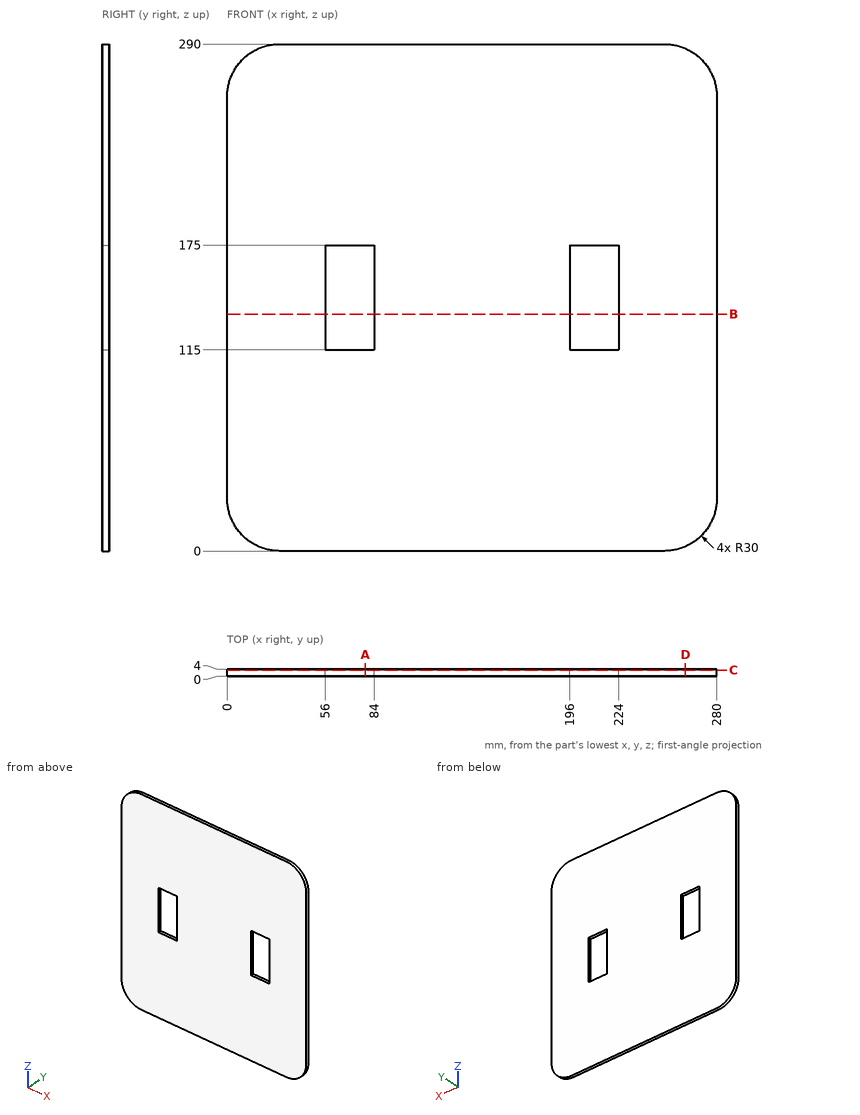
Study the drawing (mm; zero at the part's minimum x, y, z) and answer. Give positions to 0.01 mm unless a question says otherwise; leave off trailing zeros. Write each loop counter-clockwise with the first axis right and the second up, starting at its lowest first coordinate (ties: lowest second). Pieces come first, ordered by that corner, then holes. Notation, with made-up numbers: (80, -30.5) -> (104, -30.5) arc R35 cw to (104, 4.5) -> close; hole circle Ø7 at (37, 79). An arc over 180 degrees is marked (long way). Write item = value, one per line. Start each with the question number.
1) The part is cut by section D-D, the plane x = 262. Determine the outline of the cut face in (y, z), and give its area (3 significant figures).
2) Straight lines are drawn through the part: line 1 along X through (y, z) = (1.25, 123); line 2 along Z through (x, y) = (219.5, 2.2); line 3 along X through (y, z) = (0.75, 275.5). For each, find the intervals that lie inside material, in ascending order.
3) The part is cut by section A-A, the plane x = 79. Determine the outline of the cut face in (y, z).
4) The part is cut by section C-C, the plane y = 3.35. Determine the outline of the cut face in (x, z), and give its area (3 significant figures).
5) The part is cut by section B-B, the plane z = 135.5. Determine the outline of the cut face in (x, y).
6) This flat-tipped pin is pushed along its axis until it touches: pin 1 (1.5 mm diameter, centred on y = 1, z = 74, fed in from -X). Where does it stop, or does it pass through?
Solutions:
q1.outline = (0, 2.5) -> (4, 2.5) -> (4, 287.5) -> (0, 287.5) -> close
q1.area = 1,140 mm²
q2.line_1 = 0 to 56, 84 to 196, 224 to 280
q2.line_2 = 0 to 115, 175 to 290
q2.line_3 = 4.31 to 275.69
q3.outline = (0, 0) -> (4, 0) -> (4, 115) -> (0, 115) -> close; (0, 175) -> (4, 175) -> (4, 290) -> (0, 290) -> close
q4.outline = (0, 30) arc R30 ccw to (30, 0) -> (250, 0) arc R30 ccw to (280, 30) -> (280, 260) arc R30 ccw to (250, 290) -> (30, 290) arc R30 ccw to (0, 260) -> close; hole (56, 115) -> (84, 115) -> (84, 175) -> (56, 175) -> close; hole (196, 115) -> (224, 115) -> (224, 175) -> (196, 175) -> close
q4.area = 77,100 mm²
q5.outline = (0, 0) -> (56, 0) -> (56, 4) -> (0, 4) -> close; (84, 0) -> (196, 0) -> (196, 4) -> (84, 4) -> close; (224, 0) -> (280, 0) -> (280, 4) -> (224, 4) -> close
q6.pin_1 = 0
